Autodesk Inventor part; units mm, degrees
ref_plane "YZ Plane" through (0, 0, 0) normal (1, 0, 0) x (0, 1, 0)
ref_plane "XZ Plane" through (0, 0, 0) normal (0, 1, 0) x (-1, 0, 0)
ref_plane "XY Plane" through (0, 0, 0) normal (0, 0, 1) x (1, 0, 0)
sketch "Sketch1" plane through (0, 0, 0) normal (0, 0, 1) x (1, 0, 0)
  line L0 (0, 0) -> (415, 0)
  line L1 (415, 0) -> (415, 86)
  line L2 (415, 86) -> (0, 86)
  line L3 (0, 86) -> (0, 0)
  line L4 (82, 32) -> (95, 32)
  line L5 (95, 32) -> (95, 20.5)
  line L6 (95, 20.5) -> (82, 20.5)
  line L7 (82, 20.5) -> (82, 32)
  line L8 (52, 32) -> (64, 32)
  line L9 (64, 32) -> (64, 15)
  line L10 (64, 15) -> (52, 15)
  line L11 (52, 15) -> (52, 32)
  circle A0 centre (140, 41) radius 11
  dimension "d0" = 415
  dimension "d1" = 86
  dimension "d2" = 82
  dimension "d3" = 54
  dimension "d4" = 13
  dimension "d5" = 11.5
  dimension "d8" = 18
  dimension "d9" = 12
  dimension "d10" = 17
  dimension "d11" = 54
  dimension "d12" = 22
  dimension "d13" = 45
  dimension "d14" = 45
ref_plane "Work Plane1" through (0, 0, 0) normal (0, 0, -1) x (-1, 0, 0)
extrude "Extrusion2" add sketch "Sketch1" along normal blind 8
hole "Hole1" at (140, 41, 8) direction (0, 0, -1) diameter 29 depth 4 tip angle 118
properties part number "placa laterala usb"
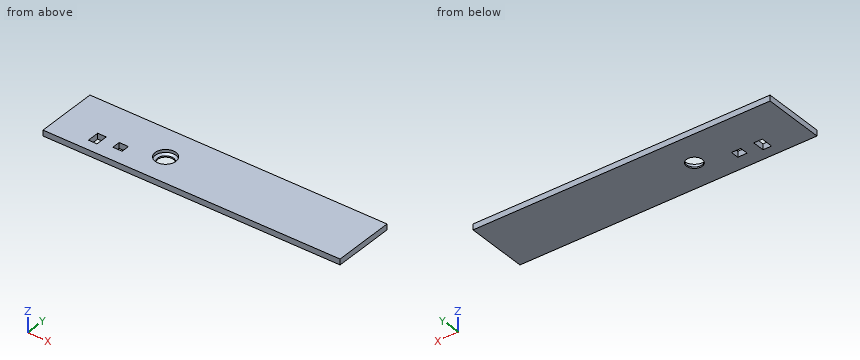
Here's how the part is built. I have some questions about the finished solid (model axes, mm). Give positions to 0.01 mm unless a question says otherwise; leave off trailing zeros. Order: outer loops, then holes, each group sorted by start corner. A loop starts at its lowest first (then second) coordinate and runs counter-clockwise, first axis right, second up. Notation, with made-up numbers: M 53.25,-15.5 L 95.25,-15.5 A28 ccw 95.25,6.5 Z; hole C 21,31.5 d8. An arc over 180 degrees is marked long. Answer as a JSON object with one key per item and string values. Group by question number.
1) Suppose I cut it at B-B, the plane y = 41. Write out the boundary of the cut face in (x, z).
2) Suppose I cut it at A-A, the plane x = 140. Write out the boundary of the cut face in (y, z).
3) Please list where these lines run through material, in increasing order: L1, parallel to Y at x = 140, z = 6.05; L2, parallel to Y at x = 140, z = 0.5; L3, parallel to X at y = 17, z = 4. Write a range as [from, to].
Results found:
{
 "1": {"outline": "M 0,0 L 129,0 L 129,1.9 L 125.5,4 L 125.5,8 L 0,8 Z; M 151,0 L 415,0 L 415,8 L 154.5,8 L 154.5,4 L 151,1.9 Z"},
 "2": {"outline": "M 0,0 L 30,0 L 30,1.9 L 26.5,4 L 26.5,8 L 0,8 Z; M 52,0 L 86,0 L 86,8 L 55.5,8 L 55.5,4 L 52,1.9 Z"},
 "3": {"L1": "[0, 26.5], [55.5, 86]", "L2": "[0, 30], [52, 86]", "L3": "[0, 52], [64, 415]"}
}
